Source: three-view drawing plus pictorial views. Frame: mm from the lowest corner of the part. Coordinates: 2 decimals unless noted, no trailing zeros. Loops run counter-clockwise (first coordinate to the right, second up) from the corner with the lowest first, then second, coordinate; pieces in that order, holes last. Notation, with made-up numbers: (7, -37.5) -> (59, -37.5) arc R14 ccw to (59, -33.5) -> close; hole circle Ø11 at (35, 39.25). An arc over 180 degrees is marked (long way). Answer as a JSON object with one key per item and string values. Group by question number.
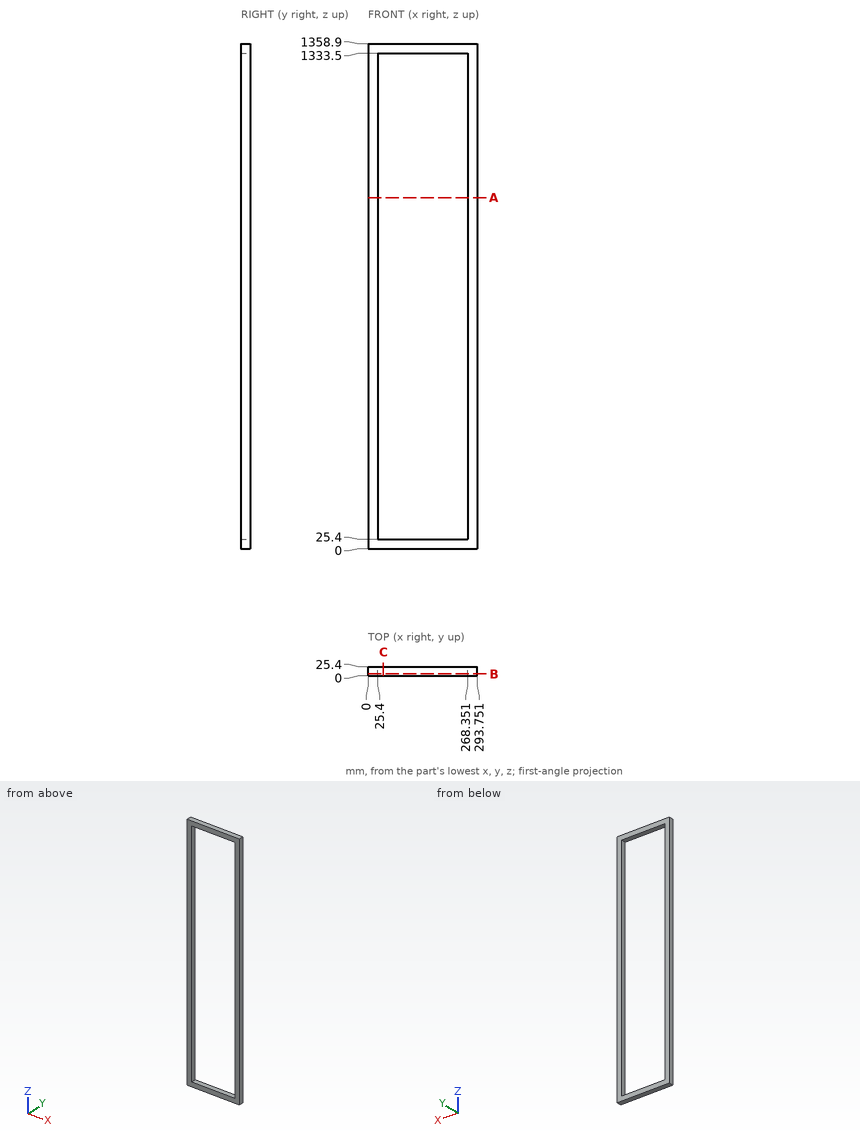
1. Section query A-A on z = 945. Return loops of the section in (x, y), then the cut area to 3 significant figures.
2. Section query C-C on x = 41. Return loops of the section in (y, z).
3. Section query B-B on y = 5.5. Return loops of the section in (x, z), then the cut area to 3 significant figures.
4. Ray query, L1, parallel to Z at x = 150.5, y = 2; L2, parallel to X at y = 8.5, z = 1192.5. Return the intervals inside material, ascending.
Solved:
{
 "1": {"outline": "(0, 0) -> (25.4, 0) -> (25.4, 25.4) -> (0, 25.4) -> close; (268.35, 0) -> (293.75, 0) -> (293.75, 25.4) -> (268.35, 25.4) -> close", "area": "1,290 mm^2"},
 "2": {"outline": "(0, 0) -> (25.4, 0) -> (25.4, 25.4) -> (0, 25.4) -> close; (0, 1333.5) -> (25.4, 1333.5) -> (25.4, 1358.9) -> (0, 1358.9) -> close"},
 "3": {"outline": "(0, 0) -> (293.75, 0) -> (293.75, 1358.9) -> (0, 1358.9) -> close; hole (25.4, 25.4) -> (268.35, 25.4) -> (268.35, 1333.5) -> (25.4, 1333.5) -> close", "area": "81,400 mm^2"},
 "4": {"L1": "0 to 25.4, 1333.5 to 1358.9", "L2": "0 to 25.4, 268.35 to 293.75"}
}
